Can you work these out from the model? Positions are in its coordinate system, mm. A direction names the side the tool comes from. Coordinates: 2 decimals unless noted, no trailing zeros. Order: outer loops, then holes, each group sorted by start corner. A loop starts at its lowest first (then second) coordinate and runs counter-clockwise, first axis right, second up. Notation, with made-up numbers: (71, 8) -> (91, 8) arc R26 ccw to (91, 30) -> close; hole circle Ø2 at (57.5, 88.5). An arc over 180 degrees is marked (long way). Use a Markdown table: item, result. Add a question column.
1. If I drill on line 1 along Z through (x, y) = (43, 3.6); line 2 along X through (y, z) = (0.4, 92); line 3 along Z through (x, y) = (-48.5, 1.5), over which ranges is the centre line in solid material (lowest first)? Write a range as from..to.
2. For pin 1 Ø1.9 at (y, z) = (3, -132) entering from -X; pin 2 Ø1.9 at (y, z) = (1.5, -106.5) entering from -X; pin 3 Ø1.9 at (y, z) = (1, -128.5) entering from -X, each with a flat end and sliding along its axis, tell me the tip position at first contact or that it passes through.
3. Suppose I cut it at C-C, the plane y = 2.8. State how many separate pieces and enclosed holes the cut face has, then the cut area to 3 significant figures.
4. Suppose I cut it at A-A, the plane z = 19. List the corners of the cut face in (x, y) for me, then the cut area to 3 significant figures.
5. Suppose I cut it at D-D, the plane z = -118. List the corners of the cut face in (x, y) for me.
6. Suppose I cut it at B-B, the plane z = -81.5. List the corners of the cut face in (x, y) for me, then the cut area to 3 significant figures.
7. For faces 1 (the flat face through (-62.224, 1.878, -36.525)), 2 (the flat face through (-129.474, 1.878, -77.988)), which set-ups out of +Z, -Z, +X, -X, +Y, -Y let a thin tool reach every point of the face, with its end or its side?
8. We'd pull the mould along X, two halves only. Please class faces 3 (the flat face through (-2, 3.81, -2)), 4 (the flat face through (126.1, 1.9, 72.4)), 5 (the flat face through (-66.3, 1.88, -30.08)): pulls with the +X half, pulls with the -X half, needs draft (parallel to the pull), parting line crosses it, or undercut.
```python
from build123d import *

# Parameters (mm, degrees)
SKETCH1_R           = 5.08
SKETCH1_R_2         = 3.81
SKETCH1_R_3         = 2.54
SKETCH1_R_4         = 1.905
SKETCH1_R_5         = 6.604
SKETCH1_W           = 21.59
SKETCH1_H           = 12.065
SKETCH1_W_2         = 50.8
SKETCH1_H_2         = 7.62
BOSS_EXTRUDE1_DEPTH = 3.81


with BuildPart() as part:
    # Sketch1 → Boss-Extrude1 (new body)
    with BuildSketch(Plane(origin=(0, 0, 0), x_dir=(1, 0, 0), z_dir=(0, 1, 0))):
        Polygon((82.300886423, -148.264316793), (171.200886423, 5.715), (88.9, 148.264316793), (-88.9, 148.264316793), (-171.200886423, 5.715), (-82.300886423, -148.264316793), align=None)
        with Locations(Location((0, -116.514316793, 0), (0, 0, 90))):
            Circle(SKETCH1_R, mode=Mode.SUBTRACT)
        with Locations(Location((-19.658728346, -139.347010207, 0), (0, 0, 90))):
            Circle(SKETCH1_R_2, mode=Mode.SUBTRACT)
        with Locations(Location((19.711271654, -139.347010207, 0), (0, 0, 90))):
            Circle(SKETCH1_R_2, mode=Mode.SUBTRACT)
        with Locations(Location((-95.25, -37.774316793, 0), (0, 0, 90))):
            Circle(SKETCH1_R_3, mode=Mode.SUBTRACT)
        with Locations(Location((95.25, -37.774316793, 0), (0, 0, 90))):
            Circle(SKETCH1_R_3, mode=Mode.SUBTRACT)
        with Locations(Location((-31.113749598, 99.396218431, 0), (0, 0, 90))):
            Circle(SKETCH1_R_4, mode=Mode.SUBTRACT)
        with Locations(Location((-33.02, -25.074316793, 0), (0, 0, 90))):
            Circle(SKETCH1_R_4, mode=Mode.SUBTRACT)
        with Locations(Location((99.06, -12.374316793, 0), (0, 0, 90))):
            Circle(SKETCH1_R_4, mode=Mode.SUBTRACT)
        with Locations(Location((99.06, 58.745683207, 0), (0, 0, 90))):
            Circle(SKETCH1_R_4, mode=Mode.SUBTRACT)
        with Locations(Location((0, 127.944316793, 0), (0, 0, 90))):
            Circle(SKETCH1_R_3, mode=Mode.SUBTRACT)
        with Locations(Location((-109.153250218, -61.114658396, 0), (0, 0, 90))):
            Circle(SKETCH1_R_3, mode=Mode.SUBTRACT)
        with Locations(Location((109.153250218, -61.114658396, 0), (0, 0, 90))):
            Circle(SKETCH1_R_3, mode=Mode.SUBTRACT)
        with Locations(Location((117.245502559, 68.866615534, 0), (0, 0, 90))):
            Circle(SKETCH1_R_5, mode=Mode.SUBTRACT)
        Polygon((-39.37, 123.785885114), (-39.37, 130.072385114), (-62.2935, 130.072385114), (-62.2935, 134.644385114), (-64.7065, 134.644385114), (-64.7065, 130.072385114), (-87.63, 130.072385114), (-87.63, 123.785885114), align=None, mode=Mode.SUBTRACT)
        Polygon((39.37, 124.039885114), (39.37, 130.326385114), (62.2935, 130.326385114), (62.2935, 134.898385114), (64.7065, 134.898385114), (64.7065, 130.326385114), (87.63, 130.326385114), (87.63, 124.039885114), align=None, mode=Mode.SUBTRACT)
        Polygon((125.416983138, -25.040114979), (130.861251839, -28.183364979), (142.323001839, -8.331031636), (146.282469985, -10.617031636), (147.488969985, -8.527312336), (143.529501839, -6.241312336), (154.991251839, 13.611021007), (149.546983138, 16.754271007), align=None, mode=Mode.SUBTRACT)
        Polygon((86.046983138, -93.230955273), (91.491251839, -96.374205273), (80.029501839, -116.226538617), (83.988969985, -118.512538617), (82.782469985, -120.602257916), (78.823001839, -118.316257916), (67.361251839, -138.16859126), (61.916983138, -135.02534126), align=None, mode=Mode.SUBTRACT)
        Polygon((-61.916983138, -135.02534126), (-67.361251839, -138.16859126), (-78.823001839, -118.316257916), (-82.782469985, -120.602257916), (-83.988969985, -118.512538617), (-80.029501839, -116.226538617), (-91.491251839, -96.374205273), (-86.046983138, -93.230955273), align=None, mode=Mode.SUBTRACT)
        Polygon((-125.416983138, -25.040114979), (-130.861251839, -28.183364979), (-142.323001839, -8.331031636), (-146.282469985, -10.617031636), (-147.488969985, -8.527312336), (-143.529501839, -6.241312336), (-154.991251839, 13.611021007), (-149.546983138, 16.754271007), align=None, mode=Mode.SUBTRACT)
        with Locations((63.5, 60.951816793)):
            Rectangle(SKETCH1_W, SKETCH1_H, mode=Mode.SUBTRACT)
        Polygon((83.059245107, 39.739198978), (72.264245107, 21.04171051), (82.712841604, 15.00921051), (93.507841604, 33.706698978), align=None, mode=Mode.SUBTRACT)
        with Locations((-63.5, 60.951816793)):
            Rectangle(SKETCH1_W, SKETCH1_H, mode=Mode.SUBTRACT)
        Polygon((-72.264245107, 21.04171051), (-83.059245107, 39.739198978), (-93.507841604, 33.706698978), (-82.712841604, 15.00921051), align=None, mode=Mode.SUBTRACT)
        Polygon((-19.559245107, -70.246027303), (-30.007841604, -76.278527303), (-19.212841604, -94.976015771), (-8.764245107, -88.943515771), align=None, mode=Mode.SUBTRACT)
        Polygon((19.559245107, -70.246027303), (8.764245107, -88.943515771), (19.212841604, -94.976015771), (30.007841604, -76.278527303), align=None, mode=Mode.SUBTRACT)
        Polygon((-0.508, -81.661), (-4.257064156, -60.399000612), (-11.761299234, -61.722199726), (-8.012235078, -82.984199114), align=None, mode=Mode.SUBTRACT)
        Polygon((4.257064156, -60.399000612), (0.508, -81.661), (8.012235078, -82.984199114), (11.761299234, -61.722199726), align=None, mode=Mode.SUBTRACT)
        Polygon((71.467492466, 41.590272297), (52.770003998, 30.795272297), (56.580003998, 24.19615872), (75.277492466, 34.99115872), align=None, mode=Mode.SUBTRACT)
        Polygon((49.858000612, 38.795935844), (71.12, 42.545), (69.796800886, 50.049235078), (48.534801499, 46.300170922), align=None, mode=Mode.SUBTRACT)
        Polygon((-71.356016539, 42.952508085), (-50.094017152, 39.203443929), (-48.770818038, 46.707679007), (-70.032817426, 50.456743163), align=None, mode=Mode.SUBTRACT)
        Polygon((-53.006020537, 31.202780382), (-71.703509005, 41.997780382), (-75.513509005, 35.398666806), (-56.816020537, 24.603666806), align=None, mode=Mode.SUBTRACT)
        with Locations((0, 107.315)):
            Rectangle(SKETCH1_W_2, SKETCH1_H_2, mode=Mode.SUBTRACT)
        with Locations((41.224971045, -30.426673737)):
            Rectangle(SKETCH1_W_2, SKETCH1_H_2, mode=Mode.SUBTRACT)
    extrude(amount=BOSS_EXTRUDE1_DEPTH)


solid = part.part
```
Worked out:
| question | item | result |
|---|---|---|
| 1 | line 1 | z = -148.26..-130.33, -124.04..26.62, 34.24..148.26 |
| 1 | line 2 | x = -114.79..-20.93, -14.06..14.06, 20.93..114.79 |
| 1 | line 3 | z = -148.26..-130.07, -123.79..148.26 |
| 2 | pin 1 | stops at x = -98.84 |
| 2 | pin 2 | stops at x = -113.56 |
| 2 | pin 3 | stops at x = -100.86 |
| 3 | separate pieces | 1 |
| 3 | enclosed holes | 33 |
| 3 | area | 70,400 mm² |
| 4 | outline | (-156.93, 0) -> (-136.16, 0) -> (-136.16, 3.81) -> (-156.93, 3.81) -> close; (-128.9, 0) -> (128.9, 0) -> (128.9, 3.81) -> (-128.9, 3.81) -> close; (136.16, 0) -> (156.93, 0) -> (156.93, 3.81) -> (136.16, 3.81) -> close |
| 4 | area | 1,140 mm² |
| 5 | outline | (-106.37, 0) -> (106.37, 0) -> (106.37, 3.81) -> (-106.37, 3.81) -> close |
| 6 | outline | (-127.45, 0) -> (127.45, 0) -> (127.45, 3.81) -> (-127.45, 3.81) -> close |
| 6 | area | 971 mm² |
| 7 | face 1 | +Y, -Y |
| 7 | face 2 | -Z, -X, +Y, -Y |
| 8 | face 3 | needs draft |
| 8 | face 4 | pulls with the +X half |
| 8 | face 5 | undercut |
